from build123d import *

# Parameters (mm, degrees)
SKETCH1_R           = 1.4
BOSS_EXTRUDE1_DEPTH = 5
CUT_EXTRUDE1_DEPTH  = 23.113344387
FILLET1_R           = 0.5


with BuildPart() as part:
    # Sketch1 → Boss-Extrude1 (new body)
    with BuildSketch(Plane(origin=(0, 0, 0), x_dir=(1, 0, 0), z_dir=(0, 1, 0))):
        Polygon((-20, 8), (20, 8), (20, 0), (14, 0), (19.75, -5), (4.25, -5), (10, 0), (-10, 0), (-4.25, -5), (-19.75, -5), (-14, 0), (-20, 0), align=None)
        with Locations(Location((12, 3, 0), (0, 0, 270))):
            Circle(SKETCH1_R, mode=Mode.SUBTRACT)
        with Locations(Location((-12, 3, 0), (0, 0, 90))):
            Circle(SKETCH1_R, mode=Mode.SUBTRACT)
        Polygon((12.476024935, 0), (11.523975065, 0), (6.923975065, -4), (17.076024935, -4), align=None, mode=Mode.SUBTRACT)
        Polygon((-12.476024935, 0), (-11.523975065, 0), (-6.923975065, -4), (-17.076024935, -4), align=None, mode=Mode.SUBTRACT)
    extrude(amount=BOSS_EXTRUDE1_DEPTH)

    # Sketch2 → Cut-Extrude1 (cut, through all)
    with BuildSketch(Plane(origin=(0, 5, 0), x_dir=(1, 0, 0), z_dir=(0, 1, 0))):
        with BuildLine():
            Line((-4.25, 0), (4.25, 0))
            ThreePointArc((4.25, 0), (0, 4.25), (-4.25, 0))
        make_face()
    extrude(amount=-CUT_EXTRUDE1_DEPTH, mode=Mode.SUBTRACT)

    # Fillet1
    fillet1_edges = [part.edges().sort_by_distance(p)[0] for p in [
        (20, 2.5, 0),
        (19.75, 2.5, 5),
        (4.25, 2.5, 5),
        (-4.25, 2.5, 5),
        (-19.75, 2.5, 5),
        (-20, 2.5, 0),
        (11.523975065, 2.5, 0),
        (12.476024935, 2.5, 0),
        (-12.476024935, 2.5, 0),
        (-11.523975065, 2.5, 0),
        (-4.25, 2.5, 0),
        (4.25, 2.5, 0),
    ]]
    fillet(fillet1_edges, radius=FILLET1_R)


solid = part.part
Read the model definition and answer for the solid it produces. Units are mm, in the model's axes. A direction names the side the tool comes from. Round coordinates to 2 decimals unless told otherwise and drop trailing zeros. Loops run counter-clockwise (first coordinate to the right, second up) from the corner with the lowest first, then second, coordinate; pieces in that order, holes last. Notation, with made-up numbers: (51, 32.5) - (72, 32.5) arc R26 cw to (72, 59.5) - close; hole circle Ø3 at (-10.75, 86). An arc over 180 degrees is marked (long way). One line per question, with ' | ' between items. Start each with the question number.
Q1. Section A-A on z = -3 is taken. Give the vertices of the cut face in (x, y).
Q2. Section B-B on x = 15.5 is taken. Give the vertices of the cut face in (y, z), plus the area to 3 significant figures.
Q3. For a pull along X with two mould halves and no side action, classify faces 4 (the flat face through (-12, 2, 4)), 5 (the flat face through (0.3, 0, -4.5)), 6 (the flat face through (16.3, 2.5, 2)) as +X half, -X half, draft (parallel to the pull), parting line (faces both ways), or undercut.
Q4. Flat-ended cylindrical pins translate along their axes: pin 1 (1.5 mm diameter, centred on y = 3.5, z = 2.5, fed in from +X); pin 2 (6 mm diameter, centred on x = -14.5, z = -0.5, fed in from -Y); pin 3 (1.7 mm diameter, centred on x = 12, z = -3, fed in from +Y). Find the tip coordinate at first contact, or state that the pin passes through.
Q5. Section C-C on y = 1.1 is taken. Count the separate pieces of the cut face and the enclosed holes in it, plus the area to 3 significant figures.
Q6. Find the intervals of material crossed by L1, parallel to Z at x = -12, y = 3.7; L2, parallel to X at y = 3.4, z = -3; L3, parallel to Z at x = -14.5, y = 3.85, in increasing order.
Q7. For faces 1 (the flat face through (17, 2, 0)), 2 (the flat face through (7.596, 2.465, 2.09)), 3 (the flat face through (-17, 2, 0)), determine the directions among +Z, -Z, +X, -X, +Y, -Y from which every point of the face is accessible in a straight line to the end or side of a thin tool.
Q8. Section D-D on x = 1 is taken. Give the vertices of the cut face in (y, z).
Established:
1) outline: (-20, 0) - (-13.4, 0) - (-13.4, 5) - (-20, 5) - close; (-10.6, 0) - (-3.01, 0) - (-3.01, 5) - (-10.6, 5) - close; (3.01, 0) - (10.6, 0) - (10.6, 5) - (3.01, 5) - close; (13.4, 0) - (20, 0) - (20, 5) - (13.4, 5) - close
2) outline: (0, -8) - (5, -8) - (5, 0) - (0, 0) - close; (0, 1.3) - (5, 1.3) - (5, 2.63) - (0, 2.63) - close; (0, 4) - (5, 4) - (5, 5) - (0, 5) - close | area: 51.6 mm²
3) face 4: undercut | face 5: draft | face 6: +X half
4) pin 1: x = 17.74 | pin 2: y = 0 | pin 3: through
5) separate pieces: 1 | enclosed holes: 4 | area: 331 mm²
6) L1: -8 to -4.4, -1.6 to 0, 4 to 5 | L2: -20 to -13.4, -10.6 to -3.01, 3.01 to 10.6, 13.4 to 20 | L3: -8 to 0, 0.43 to 1.76, 4 to 5
7) face 1: +X, +Y, -Y | face 2: +Y, -Y | face 3: -X, +Y, -Y
8) outline: (0, -8) - (5, -8) - (5, -4.13) - (0, -4.13) - close
